Source: CAD feature listing. Evaluate the final solid. Frame: model axes, mm. Face numbers are marked on the shaded views. Round coordinates to 2 decimals unless told otherwise and drop trailing zeros. Order: outer loops, then holes, each group sorted by start corner. A loop starts at its lowest first (then second) coordinate and runs counter-clockwise, first axis right, second up. Notation, with made-up numbers: (7, -10) - (41, -10) arc R17 cw to (41, 11) - close; hole circle Ø11 at (77.5, -39.5). An arc over 180 degrees is marked (long way). Return JSON: item names as keys, results as strings. Group by question number.
1) Contact query for flat-ended pins moving along their axis: P1, Ø1.5, axis at x = -17, y = 11.5, coming from the -Z side; P2, Ø3, axis at x = -11, y = -18, coming from the +Z side; P3, Ø8, axis at x = -10, y = 19, coming from the -Z side; P4, Ø1, axis at x = -29, z = 1, coming from the +Y side. Output: stop coordinate, or through.
2) Mould query, pull axis Y, two halves, no side actions, for the marked faces 1, 2 and 3. Classes: pulls with the +Y half, pulls with the -Y half, needs draft (parallel to the pull), parting line crosses it, or undercut.
3) Section A-A, the plane z = 5.75. Return loops of the section in (x, y), plus the area to 3 significant figures.
4) Ray query, line 1 (X direction, y = 30.5, z = 2.25); line 2 (Y direction, x = -28, z = 3); line 3 (X direction, y = 25.5, z = 2.25). Return the intervals inside material, ascending. Write a range as from..to.
```python
from build123d import *

# Parameters (mm, degrees)
F0_R     = 11.0998
F1_DEPTH = 6.9342
F2_SIZE  = 3.4671
F3_SIZE  = 3.46709


# Not quite as in the source:
# - a fillet or chamfer is up to 0.001 mm smaller than in the source, because OpenCascade refuses the exact size


with BuildPart() as f1:
    # F0 (on Top) → F1 (new body)
    with BuildSketch(Plane.XY):
        Polygon((12.7, 13.7528510513), (0, 45.72), (-12.7, 13.7528510513), (-45.72, 0), (-12.7, -11.6471489487), (0, -45.72), (12.7, -11.6471489487), (45.72, 0), align=None)
        Circle(F0_R, mode=Mode.SUBTRACT)
    extrude(amount=F1_DEPTH)

    # F2
    f2_edges = [f1.edges().sort_by_distance(p)[0] for p in [
        (6.35, -28.683574, 6.9342),
        (29.21, -5.823574, 6.9342),
        (-29.21, -5.823574, 6.9342),
        (-6.35, 29.736426, 6.9342),
        (-29.21, 6.876426, 6.9342),
        (6.35, 29.736426, 6.9342),
        (29.21, 6.876426, 6.9342),
        (-6.35, -28.683574, 6.9342),
    ]]
    chamfer(f2_edges, length=F2_SIZE)

    # F3 (size 3.4671 in the source; OpenCascade refuses exactly that, so slightly less here)
    f3_edges = [f1.edges().sort_by_distance(p)[0] for p in [
        (6.35, -28.683574, 0),
        (29.21, -5.823574, 0),
        (-29.21, -5.823574, 0),
        (-6.35, -28.683574, 0),
        (6.35, 29.736426, 0),
        (29.21, 6.876426, 0),
        (-29.21, 6.876426, 0),
        (-6.35, 29.736426, 0),
    ]]
    chamfer(f3_edges, length=F3_SIZE)


solid = f1.part
```
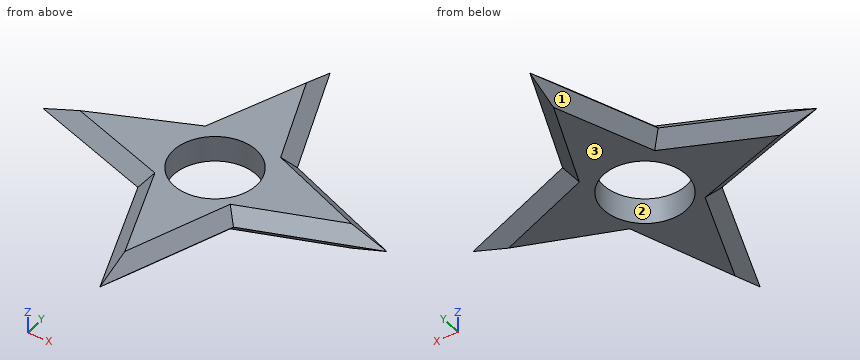
Geometry check:
{
 "1": {"P1": "z = 2.29", "P2": "z = 4.34", "P3": "z = 0", "P4": "y = 4.87"},
 "2": {"face 1": "pulls with the +Y half", "face 2": "undercut", "face 3": "needs draft"},
 "3": {"outline": "(-39.36, 0.18) - (-10.93, -9.85) - (0, -39.18) - (10.93, -9.85) - (39.36, 0.18) - (10.93, 12.02) - (0, 39.54) - (-10.93, 12.02) - close; hole circle Ø22.2 at (0, 0)", "area": "1,330 mm2"},
 "4": {"line 1": "-4.74..4.74", "line 2": "-5.76..6.87", "line 3": "-6.72..6.72"}
}
